Source: CAD feature listing. Evaluate the final solid. Frame: model axes, mm. Face numbers are marked on the shaded views. A direction names the side the tool comes from. Give positions to 0.01 mm unless a question says otherwise; leave off trailing zeros. Write each loop counter-clockwise with the first axis right and the second up, starting at its lowest first coordinate (ties: lowest second). Pieces come first, ordered by that corner, then holes. Notation, with made-up numbers: (76.25, 85.25) -> (118.25, 85.25) arc R23 ccw to (118.25, 113.25) -> close; hole circle Ø6 at (42.5, 64.25). An arc over 180 degrees is marked (long way). Answer as a JSON object with one key per item and string values. Group by question number.
Item 1: Section query B-B on x = 0. Give the number of separate pieces and of enclosed holes in the cut face, plus the area to 3 significant figures.
Item 2: Section query D-D on z = 3.25. Return the cut outline in (x, y).
Item 3: First-contact query: pin 1 Ø1 at (x, z) = (6, 5.5) entering from +Y; pin 2 Ø1.8 at (x, y) = (-8, 0) entering from +Z; pin 3 Ø3 at (x, z) = (0, 7.2) entering from -Y; pin 4 Ø4 at (y, z) = (4, 7.5) entering from +X. Flat tips, straight axial feed; report the tip coordinate or a pass-through.
Item 4: Access query for the marked faces 5 and 6. Directions: +Z, -Z, +X, -X, +Y, -Y. A direction counts if a zero-diameter tool reaches every point of the face in a straight line with its end or side. Return the directions, or none.
Item 5: Ray query, probe 1 along X at (y, z) = (0, 6.25); probe 2 along Y at (x, z) = (-8, 9.5); probe 3 along X at (y, z) = (0.25, 3.25). Return the intervals inside material, ascending. Write a range as from..to.
Item 6: Pull-direction query (X, two-part tool) for the marked faces 1, 2, 3 and 4; classes: pulls with the +X half, pulls with the -X half, needs draft (parallel to the pull), parting line crosses it, or undercut.
Item 7: Section query A-A on z = 7.2. Return the cut outline in (x, y).
Autodesk Inventor part; units mm, degrees
ref_plane "YZ Plane" through (0, 0, 0) normal (1, 0, 0) x (0, 1, 0)
ref_plane "XZ Plane" through (0, 0, 0) normal (0, 1, 0) x (-1, 0, 0)
ref_plane "XY Plane" through (0, 0, 0) normal (0, 0, 1) x (1, 0, 0)
sketch "Sketch1" plane through (0, 0, 0) normal (0, 0, 1) x (1, 0, 0)
  circle A0 centre (0, 0) radius 2.55
  circle A1 centre (0, 0) radius 10.5
  dimension "d0" = 21
  dimension "d1" = 5.1
extrude "Extrusion1" add sketch "Sketch1" along normal blind 11
sketch "Sketch3" plane through (0, 0, 0) normal (0, 0, -1) x (-1, 0, 0)
  circle A0 centre (0, 0) radius 4.5
  dimension "d12" = 9
extrude "Extrusion2" cut sketch "Sketch3" against normal blind 3
chamfer "Chamfer1" distance 1.93 angle 45 1 edges at (-2.55, 0, 3)
sketch "Sketch4" plane through (0, 0, 11) normal (0, 0, 1) x (1, 0, 0)
  line L0 (10, -8) -> (-10, -8)
  line L1 (-10, -8) -> (-10, -18)
  line L2 (-10, -18) -> (10, -18)
  line L3 (10, -18) -> (10, -8)
  point P0 (0, 0)
  point P1 (0, -8)
  dimension "d18" = 20
  dimension "d19" = 8
  dimension "d20" = 10
extrude "Extrusion3" cut sketch "Sketch4" against normal through all
sketch "Sketch2" plane through (0, 0, 11) normal (0, 0, 1) x (1, 0, 0)
  circle A0 centre (0, 0) radius 8 construction
  point P0 (-8, 0)
  point P1 (8, 0)
  dimension "d4" = 16
hole "Hole1" at (-8, 0, 11) at (8, 0, 11) direction (0, 0, -1) diameter 2.3 end through all countersink diameter 4 countersink angle 90
sketch "Sketch5" plane through (0, 0, 0) normal (1, 0, 0) x (0, 1, 0)
  line L0 (-1, 7.2) -> (-12.4416, 7.2)
  line L1 (-8, 11) -> (-8, 0)
  line L2 (-8, 9.6) -> (-3, 9.6)
  line L3 (-3, 9.6) -> (-3, 9.2)
  line L4 (-3, 9.2) -> (-2, 9.2)
  line L5 (-2.55, 11) -> (-2.55, 4.93)
  line L6 (-2, 9.2) -> (-2, 7.2)
  line L7 (-8, 9.6) -> (-8, 7.2)
  line L8 (10.5, 11) -> (-8, 11)
  point P0 (0, 0)
  dimension "d23" = 4.8
  dimension "d24" = 4
  dimension "d25" = 5
  dimension "d27" = 1.4
  dimension "d28" = 1
revolve "Revolution1" cut sketch "Sketch5" angle 360 about axis through (0, -1, 7.2) along (0, -1, 0) contours L0 L5 L4 L6 | L0 L1 L2 L3 L4 L5
chamfer "Chamfer2" distance 0.4 angle 45 8 edges at (0, 10.5, 11) (0, -8, 11) (0, 10.5, 0) (0, -8, 0) (4.5, 0, 0) (-8, 1.15, 0) (8, 1.15, 0) (-2.55, 0, 11)
properties part number "shaft-coupler-pla" material "ABS Plastic"
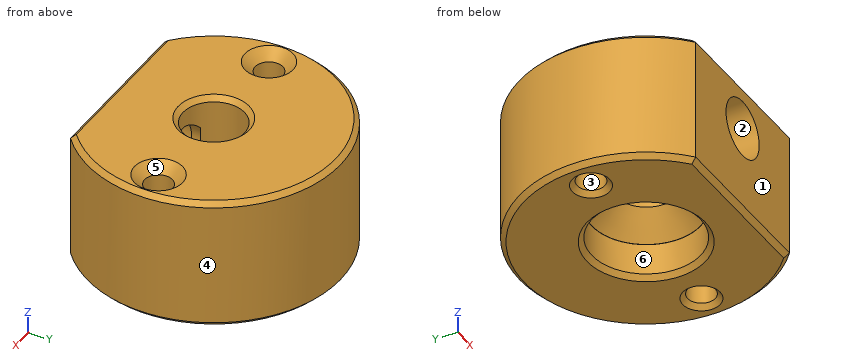
Worked answers:
{
 "1": {"separate pieces": "3", "enclosed holes": "0", "area": "106 mm^2"},
 "2": {"outline": "(-6.8, -8) -> (6.8, -8) arc R10.5 ccw (long way) to start; hole circle Ø2.3 at (-8, 0); hole circle Ø8.46 at (0, 0); hole circle Ø2.3 at (8, 0)"},
 "3": {"pin 1": "y = 8.94", "pin 2": "through", "pin 3": "y = 2.06", "pin 4": "x = 10.31"},
 "4": {"face 5": "+Z", "face 6": "-Z"},
 "5": {"probe 1": "-10.5..-9.15, -6.85..-2.55, 2.55..6.85, 9.15..10.5", "probe 2": "-6.8..-1.15, 1.15..6.8", "probe 3": "-10.5..-9.12, -6.88..-4.22, 4.22..6.88, 9.12..10.5"},
 "6": {"face 1": "needs draft", "face 2": "undercut", "face 3": "undercut", "face 4": "parting line crosses it"},
 "7": {"outline": "(-6.8, -8) -> (-2.4, -8) -> (-2.4, -3) -> (-2, -3) -> (-2, -2) -> (-1.58, -2) arc R2.55 cw (long way) to (1.58, -2) -> (2, -2) -> (2, -3) -> (2.4, -3) -> (2.4, -8) -> (6.8, -8) arc R10.5 ccw (long way) to start; hole circle Ø2.3 at (-8, 0); hole circle Ø2.3 at (8, 0)"}
}
